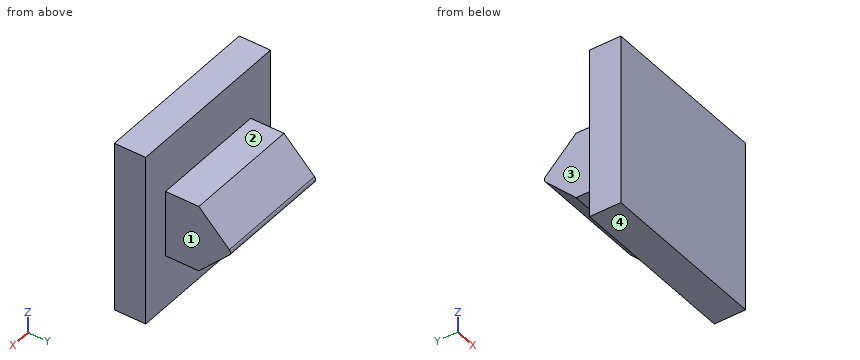
```python
from build123d import *

# Parameters (mm, degrees)
RESSALTO_EXTRUS_O1_DEPTH      = 22
RESSALTO_EXTRUS_O1_DEPTH_BACK = 22
RESSALTO_EXTRUS_O2_DEPTH      = 15
RESSALTO_EXTRUS_O2_DEPTH_BACK = 15


with BuildPart() as part:
    # Esboço2 → Ressalto-extrusão1 (new, two sides: drawn at the far end of the back side and taken through both)
    with BuildSketch(Plane.XY.offset(-RESSALTO_EXTRUS_O1_DEPTH_BACK)):
        Polygon((0, 0), (22, 0), (22, -8), (0, -8), (-22, -8), (-22, 0), align=None)
    extrude(amount=RESSALTO_EXTRUS_O1_DEPTH + RESSALTO_EXTRUS_O1_DEPTH_BACK)

    # Esboço4 → Ressalto-extrusão2 (add, two sides: drawn at the far end of the back side and taken through both)
    with BuildSketch(Plane(origin=(0, 0, 0), x_dir=(0, 0, -1), z_dir=(1, 0, 0)).offset(-RESSALTO_EXTRUS_O2_DEPTH_BACK)):
        with BuildLine():
            Line((-8.5, 8.5), (-0.707106781, 16.292893219))
            ThreePointArc((-0.707106781, 16.292893219), (0, 16.585786438), (0.707106781, 16.292893219))
            Line((0.707106781, 16.292893219), (8.5, 8.5))
            Line((8.5, 8.5), (8.5, 0))
            Line((8.5, 0), (0, 0))
            Line((0, 0), (-8.5, 0))
            Line((-8.5, 0), (-8.5, 8.5))
        make_face()
    extrude(amount=RESSALTO_EXTRUS_O2_DEPTH + RESSALTO_EXTRUS_O2_DEPTH_BACK)


solid = part.part
```
Could you check a few things on this model? Use its own coordinates, in mm. Face numbers are marked on the shaded views. A direction names the side the tool comes from. Round coordinates to 2 decimals unless told otherwise and drop trailing zeros. Loops run counter-clockwise (first coordinate to the right, second up) from the corner with the lowest first, then second, coordinate; pieces in that order, holes last.
Q1. On a 3-axis mill with a long thin cutter (end or side, diameter ignored), from which of +Z, -Z, +X, -X, +Y, -Y can I reach the whole of each face in a straight line? I mean the marked faces 1, 2, 3 and 4. Say none if no direction works.
Q2. I want a section at B-B (x = 3). Write out the boundary of the cut face in (y, z), and give its area (3 significant figures).
Q3. Please list where these lines run through material, in increasing order: L1, parallel to X at y = 10.75, z = 1; L2, parallel to Y at x = -20, z = 16.5; L3, parallel to Z at x = 5, y = 7.
Q4. I want a section at C-C (y = 9.75). Write out the boundary of the cut face in (x, z).
Q5. For P1, Ø2, axis at x = -4.5, y = 6, coming from the -Z side; P2, Ø5, axis at y = 4, z = -3.5, coming from the -X side; P3, Ø8, axis at y = 7, z = -4, coming from the +X side; P4, Ø5, axis at y = 4.5, z = -13, coming from the +X side, each with a flat end and sliding along its axis, tell me the tip position at first contact or that it passes through.
Q6. I want a section at D-D (z = 0). Write out the boundary of the cut face in (x, y), and give its area (3 significant figures).
Q7. I want a section at A-A (z = 5). Write out the boundary of the cut face in (x, y), and give its area (3 significant figures).
Answer below:
1. face 1: +Z, -Z, +X, +Y
1. face 2: +Z, +X, -X, +Y
1. face 3: +Z, -Z, -X, +Y
1. face 4: -Z, +X, -X, +Y, -Y
2. outline: (-8, -22) - (0, -22) - (0, -8.5) - (8.5, -8.5) - (16.29, -0.71) arc R1 ccw to (16.29, 0.71) - (8.5, 8.5) - (0, 8.5) - (0, 22) - (-8, 22) - close
2. area: 569 mm2
3. L1: x = -15 to 15
3. L2: y = -8 to 0
3. L3: z = -8.5 to 8.5
4. outline: (-15, -7.25) - (15, -7.25) - (15, 7.25) - (-15, 7.25) - close
5. P1: stops at z = -8.5
5. P2: stops at x = -15
5. P3: stops at x = 15
5. P4: passes through
6. outline: (-22, -8) - (22, -8) - (22, 0) - (15, 0) - (15, 16.59) - (-15, 16.59) - (-15, 0) - (-22, 0) - close
6. area: 850 mm2
7. outline: (-22, -8) - (22, -8) - (22, 0) - (15, 0) - (15, 12) - (-15, 12) - (-15, 0) - (-22, 0) - close
7. area: 712 mm2
